Here's how the part is built. I have some questions about the finished solid (model axes, mm). A direction names the side the tool comes from. Round coordinates to 2 decimals unless told otherwise and drop trailing zeros. Loops run counter-clockwise (first coordinate to the right, second up) from the corner with the lowest first, then second, coordinate; pieces in that order, holes last. Notation, with made-up numbers: M -34.75,16.25 L 18.25,16.25 A26 cw 18.25,45.25 Z; hole C 57,7 d7. An arc over 180 degrees is marked long. Answer as a JSON object with one key per item and string values.
from build123d import *

# Parameters (mm, degrees)
SKETCH_2_W             = 64.02174429
SKETCH_2_H             = 9.248919907
CUT_EXTRUDE_1_DEPTH    = 49
HOLE_WIZARD_M4_2_D     = 3.3
HOLE_WIZARD_M4_2_DEPTH = 5.5
HOLE_WIZARD_M4_2_TIP   = 0.991420021
HOLE_WIZARD_M6_2_D     = 5
HOLE_WIZARD_M6_2_DEPTH = 5.5
HOLE_WIZARD_M6_2_TIP   = 1.502151548


with BuildPart() as part:
    # 草图1 → 旋转1 (revolve)
    with BuildSketch(Plane(origin=(0, 0, 0), x_dir=(1, 0, 0), z_dir=(0, 1, 0)), mode=Mode.PRIVATE) as revolve_1_sk:
        Polygon((25.4, 7.5), (25.4, -7.5), (17, -7.5), (17, -3), (17.6, -3), (17.6, -2), (15, -2), (15, 2), (17.6, 2), (17.6, 3), (17, 3), (17, 7.5), align=None)
    revolve(revolve_1_sk.sketch.rotate(Axis((0, 0, -31.9390681), (0, 0, 1)), 180), axis=Axis((0, 0, -31.9390681), (0, 0, 1)))  # turned: the seam where the file's is

    # 草图2 → 切除-拉伸1 (cut)
    with BuildSketch(Plane.XY.offset(7.5)):
        with Locations((-1.141100508, 29.124459954)):
            Rectangle(SKETCH_2_W, SKETCH_2_H)
        with Locations((-1.141100508, -29.124459954)):
            Rectangle(SKETCH_2_W, SKETCH_2_H)
    extrude(amount=-CUT_EXTRUDE_1_DEPTH, mode=Mode.SUBTRACT)

    # M4 螺纹孔2
    with Locations(Plane(origin=(0, 24.5, 0), x_dir=(1, 0, 0), z_dir=(0, 1, 0))):
        with Locations((0, 0)):
            Hole(HOLE_WIZARD_M4_2_D / 2, depth=HOLE_WIZARD_M4_2_DEPTH)
            with Locations((0, 0, -(HOLE_WIZARD_M4_2_DEPTH + HOLE_WIZARD_M4_2_TIP / 2))):  # 118° drill point
                Cone(0, HOLE_WIZARD_M4_2_D / 2, HOLE_WIZARD_M4_2_TIP, mode=Mode.SUBTRACT)

    # M6 螺纹孔2
    with Locations(Plane(origin=(0, -24.5, 0), x_dir=(-1, 0, 0), z_dir=(0, -1, 0))):
        with Locations((0, 0)):
            Hole(HOLE_WIZARD_M6_2_D / 2, depth=HOLE_WIZARD_M6_2_DEPTH)
            with Locations((0, 0, -(HOLE_WIZARD_M6_2_DEPTH + HOLE_WIZARD_M6_2_TIP / 2))):  # 118° drill point
                Cone(0, HOLE_WIZARD_M6_2_D / 2, HOLE_WIZARD_M6_2_TIP, mode=Mode.SUBTRACT)


solid = part.part
Item 1: For faces 5 (the face through (2.213, -16.855, 5.219)), 6 (the face through (1.216, 21.712, -1.115)), 7 (the face through (-0.54, -21.71, 2.44)), 8 (the face through (13, -8, -2)), 9 (the face through (2.213, -16.855, -5.281)), which set-ups out of +Z, -Z, +X, -X, +Y, -Y let a thin tool reach every point of the face, with its end or its side?
Solution:
{"face 5": "+Z", "face 6": "+Y", "face 7": "-Y", "face 8": "none", "face 9": "-Z"}
Item 2: I want a section at B-B on y = -13. List the corners of the cut face in (x, z) for me.
Solution:
{"outline": "M -21.82,-7.5 L -10.95,-7.5 L -10.95,-3 L -11.86,-3 L -11.86,-2 L -7.48,-2 L -7.48,2 L -11.86,2 L -11.86,3 L -10.95,3 L -10.95,7.5 L -21.82,7.5 Z; M 7.48,-2 L 11.86,-2 L 11.86,-3 L 10.95,-3 L 10.95,-7.5 L 21.82,-7.5 L 21.82,7.5 L 10.95,7.5 L 10.95,3 L 11.86,3 L 11.86,2 L 7.48,2 Z"}
Item 3: If I drill on L1, parallel to Z at x = 0, y = -22.05; L2, parallel to Y at x = 0, z = -4.15; L3, parallel to Z at x = -13.5, y = -8, over which ranges is the centre line in solid material (lowest first)? Write a range as from..to.
Solution:
{"L1": "z = -7.5..-2.5, 2.5..7.5", "L2": "y = -24.5..-17, 17..24.5", "L3": "z = -2..2"}
Item 4: I want a section at A-A on x = 5.5. List the corners of the cut face in (y, z) for me, plus the area to 3 significant figures.
Solution:
{"outline": "M -24.5,-7.5 L -16.09,-7.5 L -16.09,-3 L -16.72,-3 L -16.72,-2 L -13.96,-2 L -13.96,2 L -16.72,2 L -16.72,3 L -16.09,3 L -16.09,7.5 L -24.5,7.5 Z; M 13.96,-2 L 16.72,-2 L 16.72,-3 L 16.09,-3 L 16.09,-7.5 L 24.5,-7.5 L 24.5,7.5 L 16.09,7.5 L 16.09,3 L 16.72,3 L 16.72,2 L 13.96,2 Z", "area": "267 mm2"}
Item 5: I want a section at D-D on y = 21. List the corners of the cut face in (x, z) for me, plus the area to 3 significant figures.
Solution:
{"outline": "M -14.29,-7.5 L 14.29,-7.5 L 14.29,7.5 L -14.29,7.5 Z; hole C 0,0 d3.3", "area": "420 mm2"}
Item 6: I want a section at C-C on z = 4.5. List the corners of the cut face in (x, y) for me.
Solution:
{"outline": "M -6.7,-24.5 L 6.7,-24.5 A25.4 ccw 6.7,24.5 L -6.7,24.5 A25.4 ccw Z; hole C 0,0 d34"}
Item 7: We'd pull the mould along X, two halves only. Please class faces 1 (the face through (-25.396, 0.464, 0.105)), 2 (the face through (0.3, 18.2, 0.1)), 3 (the face through (25.396, -0.464, 0.105)), 4 (the face through (0.094, -17.759, 0.424)): +X half, -X half, draft (parallel to the pull), parting line (faces both ways), or undercut.
Solution:
{"face 1": "-X half", "face 2": "undercut", "face 3": "+X half", "face 4": "undercut"}
Item 8: For P1, Ø2, axis at x = -17, z = 5, coming from the +Y side; P2, Ø4, axis at x = 0, z = 0, coming from the -Y side; P3, Ø6, axis at y = -13, z = -1, coming from the -X side; P4, Ø5, axis at x = -8, z = 0, coming from the -Y side, each with a flat end and sliding along its axis, tell me the tip position at first contact or that it passes through.
Solution:
{"P1": "stops at y = 19.73", "P2": "stops at y = -18.7", "P3": "stops at x = -23.35", "P4": "stops at y = -24.5"}
